The figure shows three views and two pictorial views of one solid part (mm, origin at its lowest corner). Answer the questions. Coordinates: 2 decimals unless noted, no trailing zeros. Loops run counter-clockwise (first coordinate to the right, second up) from the corner with the lowest first, then second, coordinate; pieces in that order, holes last. Notation, with made-up numbers: M -22.5,78.25 L 14.5,78.25 A20 ccw 14.5,85.25 Z; hole C 1,80.5 d2. An arc over 180 degrees is marked long. Write each question's results on one line, items separated by ' | '.
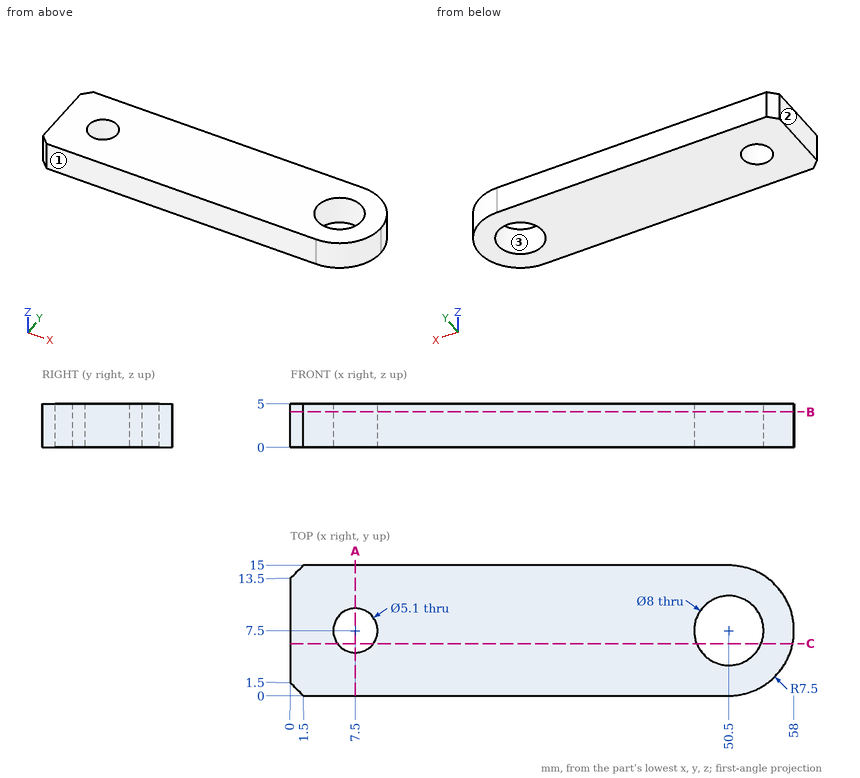
1) Find section A-A, the plane x = 7.5. Give the vertices of the cut face in (y, z), and give its area (3 significant figures).
Check result:
outline: M 0,0 L 4.95,0 L 4.95,5 L 0,5 Z; M 10.05,0 L 15,0 L 15,5 L 10.05,5 Z | area: 49.5 mm^2
2) For a pull along X with two mould halves and no side action, classify the marked faces 1, 2 and 3 as released by +X, released by -X, zero draft, split by the parting line, or undercut.
Check result:
face 1: zero draft | face 2: released by -X | face 3: undercut
3) Given pin 1 Ø1 at (y, z) = (2, 4.5) entering from +X, flat-ended and moving along its own axis, determine where the tip first touches the part or whether it passes through.
Check result:
pin 1: x = 56.09
4) Find section C-C, the plane y = 6. Give the vertices of the cut face in (x, z).
Check result:
outline: M 0,0 L 5.44,0 L 5.44,5 L 0,5 Z; M 9.56,0 L 46.79,0 L 46.79,5 L 9.56,5 Z; M 54.21,0 L 57.85,0 L 57.85,5 L 54.21,5 Z
5) Straight lines are drawn through the part: probe 1 along Y at (x, z) = (50.5, 2.05); probe 2 along Y at (x, z) = (7.5, 3.55); probe 3 along X at (y, z) = (6.25, 3.45). For each, find the intervals that lie inside material, in ascending order. Write a range as [from, to].
Check result:
probe 1: [0, 3.5], [11.5, 15] | probe 2: [0, 4.95], [10.05, 15] | probe 3: [0, 5.28], [9.72, 46.7], [54.3, 57.9]
6) Find section B-B, the plane z = 4.1. Give the vertices of the cut face in (x, y), and give its area (3 significant figures).
Check result:
outline: M 0,1.5 L 1.5,0 L 50.5,0 A7.5 ccw 50.5,15 L 1.5,15 L 0,13.5 Z; hole C 7.5,7.5 d5.1; hole C 50.5,7.5 d8 | area: 773 mm^2
